Work out the finished part from the listing and answer in its coordinate system (mm). A direction names the side the tool comes from. Give positions to 0.01 mm unless a question says otherwise; leave off trailing zeros. Write each loop counter-clockwise with the first axis right and the second up, starting at its lowest first coordinate (ties: lowest second). Pieces come first, ordered by that corner, then holes. Notation, with made-up numbers: (7.25, -3) -> (54.25, -3) arc R5 cw to (54.25, 2) -> close; hole circle Ø4 at (-35.5, -8.5). An arc over 180 degrees is marked (long way). Use a Markdown table: item, result. Add a question column.
Q1. Section C-C, the plane z = -10 is taken. Give the vertices of the cut face in (x, y).
Q2. For faces 1 (the face through (27.982, -0.49, 28.584)), 2 (the face through (-16.9, 35, -36.5)), determine the directions among +Z, -Z, +X, -X, +Y, -Y from which every point of the face is accessible in a straight line to the end or side of a thin tool.
Q3. Each of these flat-tipped pins is pushed along its axis until it touches: pin 1 Ø8 at (y, z) = (-9.5, 10.5) entering from +X; pin 2 Ø3 at (y, z) = (17, 35.5) entering from +X; pin 3 Ø8 at (x, y) = (13.5, -16) entering from +Z. Where does it stop, or does it pass through?
Q4. Consider line 1 (Z direction, x = 1.5, y = -13) (3 decimals); line 2 (X direction, y = -27.5, z = -25.5); line 3 (Z direction, x = -36, y = 23). Determine where each line is inside the solid, lowest interval first.
Q5. For a pull along Z with two mould halves and no side action, classify faces 3 (the face through (-16.9, -35, -36.5)), 4 (the face through (-28.584, -0.49, 27.982)), 5 (the face through (20.765, -0.49, -39.923)) as pulls with the +Z half, pulls with the -Z half, needs draft (parallel to the pull), parting line crosses it, or undercut.
Q6. Section B-B, the plane x = 9 is taken. Give the vertices of the cut face in (y, z).
from build123d import *

# Parameters (mm, degrees)
F0_R     = 45
F1_DEPTH = 35


with BuildPart() as f1:
    # F0 (on Front) → F1 (new body, symmetric)
    with BuildSketch(Plane.XZ):
        Circle(F0_R)
        with BuildLine():
            ThreePointArc((0.999922, 39.9875), (28.284271, 28.284271), (39.9875, 0.999922))
            ThreePointArc((39.9875, 0.999922), (40.702673, 0.711512), (41, 0))
            ThreePointArc((41, 0), (40.702673, -0.711512), (39.9875, -0.999922))
            ThreePointArc((39.9875, -0.999922), (28.284271, -28.284271), (0.999922, -39.9875))
            ThreePointArc((0.999922, -39.9875), (0.99998, -39.99375), (1, -40))
            ThreePointArc((1, -40), (-0.00625, -40.99998), (-0.999922, -39.9875))
            ThreePointArc((-0.999922, -39.9875), (-28.284271, -28.284271), (-39.9875, -0.999922))
            ThreePointArc((-39.9875, -0.999922), (-41, 0), (-39.9875, 0.999922))
            ThreePointArc((-39.9875, 0.999922), (-28.284271, 28.284271), (-0.999922, 39.9875))
            ThreePointArc((-0.999922, 39.9875), (-0.00625, 40.99998), (1, 40))
            ThreePointArc((1, 40), (0.99998, 39.99375), (0.999922, 39.9875))
        make_face(mode=Mode.SUBTRACT)
    extrude(amount=F1_DEPTH, both=True)


solid = f1.part
Result set:
| question | item | result |
|---|---|---|
| 1 | outline | (-43.87, -35) -> (-38.73, -35) -> (-38.73, 35) -> (-43.87, 35) -> close; (38.73, -35) -> (43.87, -35) -> (43.87, 35) -> (38.73, 35) -> close |
| 2 | face 1 | +Y, -Y |
| 2 | face 2 | +Z, -Z, +X, -X, +Y |
| 3 | pin 1 | stops at x = 44.53 |
| 3 | pin 2 | stops at x = 29.48 |
| 3 | pin 3 | stops at z = 43.99 |
| 4 | line 1 | z = -44.975 to -39.972, 39.972 to 44.975 |
| 4 | line 2 | x = -37.08 to -30.82, 30.82 to 37.08 |
| 4 | line 3 | z = -27 to -17.44, 17.44 to 27 |
| 5 | face 3 | needs draft |
| 5 | face 4 | undercut |
| 5 | face 5 | parting line crosses it |
| 6 | outline | (-35, -44.09) -> (35, -44.09) -> (35, -38.97) -> (-35, -38.97) -> close; (-35, 38.97) -> (35, 38.97) -> (35, 44.09) -> (-35, 44.09) -> close |
